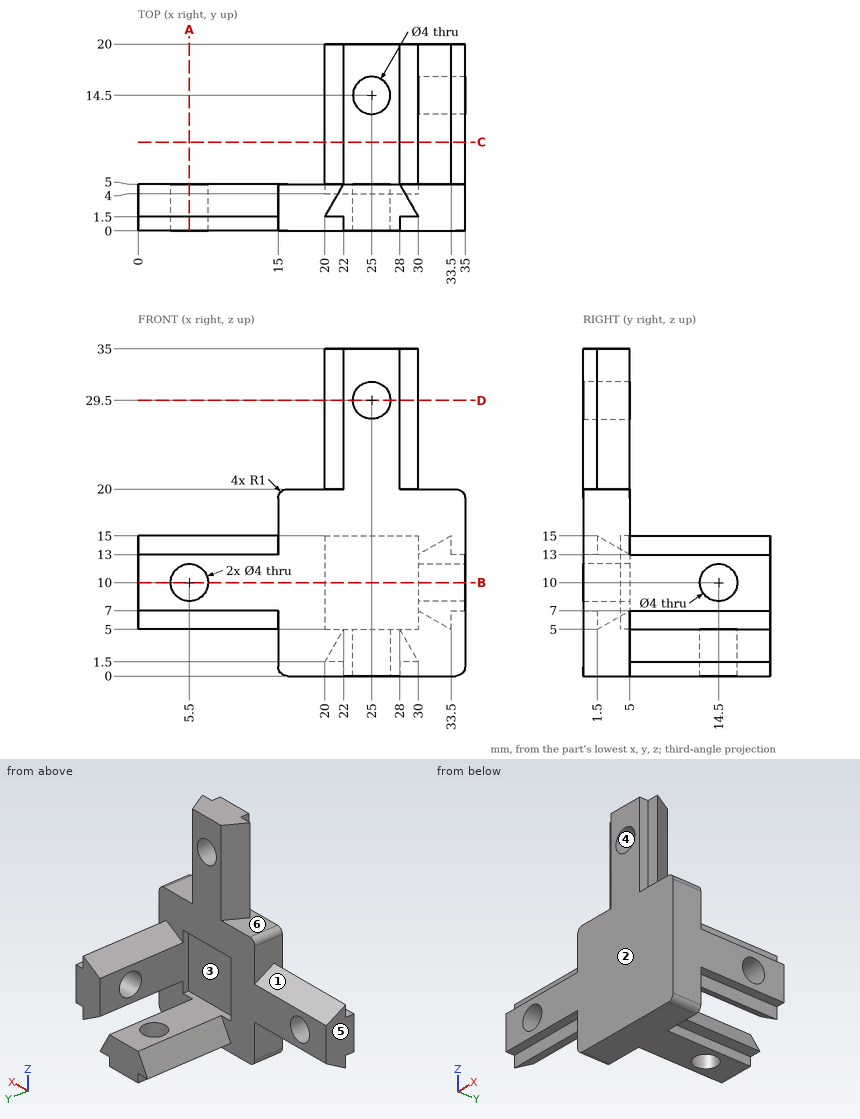
The figure shows three views and two pictorial views of one solid part (mm, origin at its lowest corner). Answer the questions. A direction names the side the tool comes from. Give positions to 0.01 mm unless a question says otherwise; leave off trailing zeros. Order: outer loops, then holes, each group sorted by start corner. A loop starts at its lowest first (then second) coordinate and runs counter-clockwise, first axis right, second up. Notation, with made-up numbers: M -16,86.25 L 16,86.25 A27 cw 16,114.25 Z; hole C 48.25,42 d7. An arc over 180 degrees is marked long. Return JSON: item names as keys, results as strings.
Q1. Each of these flat-tipped pins is pushed along its axis until it touches: pin 1 (12 mm diameter, centred on y = 3, z = 31, fed in from -X); pin 2 (11 mm diameter, centred on x = 27, z = 9.5, fed in from +Y); pin 3 (8 mm diameter, centred on x = 18.5, z = 25.5, fed in from +Y); pin 4 (5 mm diameter, centred on x = 16.5, y = 16, fed in from -Z). Where does it stop, or does it pass through?
Answer below:
{"pin 1": "stops at x = 20", "pin 2": "stops at y = 20", "pin 3": "stops at y = 5", "pin 4": "passes through"}
Q2. Find section D-D, the plane z = 29.5. Write down the section's boundary in (x, y).
Answer below:
{"outline": "M 20,1.5 L 22,1.5 L 22,0 L 23,0 L 23,5 L 22,5 Z; M 27,0 L 28,0 L 28,1.5 L 30,1.5 L 28,5 L 27,5 Z"}
Q3. Find the intervals of material crossed by line 1 along Y through (x, z) = (33.55, 10); line 2 along Z through (x, y) = (23, 18.75); line 3 along X through (y, z) = (3.75, 29.5), in increasing order. Write a range as [from, to].
Answer below:
{"line 1": "y = [0, 12.5], [16.5, 20]", "line 2": "z = [0, 5]", "line 3": "x = [21.29, 23], [27, 28.71]"}
Q4. The mould has two halves that part along X. Classify the marked faces 4, 5 and 6: pulls with the +X half, pulls with the -X half, needs draft (parallel to the pull), parting line crosses it, or undercut.
Answer below:
{"face 4": "undercut", "face 5": "pulls with the -X half", "face 6": "needs draft"}
Q5. Which of the six approach directions +Z, -Z, +X, -X, +Y, -Y give full straight-line access (tool end or side, diameter ignored) to the marked faces 1, 2 and 3?
Answer below:
{"face 1": "+Z, -X, +Y", "face 2": "+Z, -Z, +X, -X, -Y", "face 3": "+Y"}
Q6. Find section B-B, the plane z = 10. Write down the section's boundary in (x, y).
Answer below:
{"outline": "M 0,0 L 3.5,0 L 3.5,5 L 0,5 Z; M 7.5,0 L 35,0 L 35,12.5 L 30,12.5 L 30,4 L 20,4 L 20,5 L 7.5,5 Z; M 30,16.5 L 35,16.5 L 35,20 L 30,20 Z"}
Q7. Find section C-C, the plane y = 9.5. Write down the section's boundary in (x, z), and give its area (3 significant figures).
Answer below:
{"outline": "M 20,1.5 L 22,1.5 L 22,0 L 28,0 L 28,1.5 L 30,1.5 L 28,5 L 22,5 Z; M 30,7 L 33.5,5 L 33.5,7 L 35,7 L 35,13 L 33.5,13 L 33.5,15 L 30,13 Z", "area": "74.0 mm^2"}
Q8. Find section A-A, the plane x = 5.5. Write down the section's boundary in (y, z), and give its area (3 significant figures).
Answer below:
{"outline": "M 0,7 L 1.5,7 L 1.5,5 L 5,7 L 5,8 L 0,8 Z; M 0,12 L 5,12 L 5,13 L 1.5,15 L 1.5,13 L 0,13 Z", "area": "17.0 mm^2"}
